Autodesk Inventor part; units mm, degrees
ref_plane "Work Plane2" through (-14.9733, -35.8014, 0) normal (0, 0, 1) x (1, 0, 0)
ref_plane "YZ Plane" through (0, 0, 0) normal (1, 0, 0) x (0, 1, 0)
ref_plane "XZ Plane" through (0, 0, 0) normal (0, 1, 0) x (-1, 0, 0)
ref_plane "Work Plane1" through (0, 0, 6.35) normal (0, 0, 1) x (1, 0, 0)
sketch "Sketch1" plane through (0, 0, 6.35) normal (0, 0, 1) x (1, 0, 0)
  line L0 (14.9733, -35.8014) -> (14.9733, 35.8014)
  line L1 (14.9733, 35.8014) -> (-14.9733, 35.8014)
  line L2 (-14.9733, 35.8014) -> (-14.9733, -35.8014)
  line L3 (-14.9733, -35.8014) -> (14.9733, -35.8014)
  circle A0 centre (-13.81, -28.5989) radius 0.6
  circle A1 centre (-11.557, -24.257) radius 0.1524
  circle A2 centre (-9.271, -23.749) radius 0.1524
  circle A3 centre (-8.636, -22.606) radius 0.1524
  circle A4 centre (-8.636, -19.939) radius 0.1524
  circle A5 centre (-6.731, -35.3061) radius 0.1524
  circle A6 centre (-5.842, -34.1631) radius 0.1524
  circle A7 centre (-7.239, -31.8771) radius 0.1524
  circle A8 centre (-5.08, -31.7501) radius 0.1524
  circle A9 centre (-5.08, -30.8611) radius 0.1524
  circle A10 centre (-1.016, -32.6391) radius 0.1524
  circle A11 centre (-1.905, -27.9401) radius 0.1524
  circle A12 centre (-4.318, -24.892) radius 0.1524
  circle A13 centre (-5.842, -19.05) radius 0.1524
  circle A14 centre (-5.08, -21.463) radius 0.1524
  circle A15 centre (-5.08, -18.415) radius 0.1524
  circle A16 centre (-4.191, -19.939) radius 0.1524
  circle A17 centre (-4.191, -18.415) radius 0.1524
  circle A18 centre (-11.176, -17.526) radius 0.1525
  circle A19 centre (-13.014, -12.8141) radius 1.016
  circle A20 centre (-7.874, -8.382) radius 1.85
  circle A21 centre (-4.826, -17.526) radius 0.1524
  circle A22 centre (-4.572, -5.715) radius 0.1524
  circle A23 centre (-2.413, -6.35) radius 0.1524
  circle A24 centre (-1.016, -5.715) radius 0.1524
  circle A25 centre (4.953, -31.4961) radius 0.1524
  circle A26 centre (6.35, -30.6071) radius 0.1524
  circle A27 centre (6.19, -28.5989) radius 0.85
  circle A28 centre (0.254, -24.638) radius 0.1524
  circle A29 centre (1.27, -21.082) radius 0.1524
  circle A30 centre (6.604, -26.2891) radius 0.1524
  circle A31 centre (5.461, -21.717) radius 0.1524
  circle A32 centre (8.509, -32.7661) radius 0.1524
  circle A33 centre (8.636, -30.6071) radius 0.1524
  circle A34 centre (12.986, -33.8141) radius 1.016
  circle A35 centre (13.843, -30.0991) radius 0.1524
  circle A36 centre (9.017, -24.892) radius 0.1524
  circle A37 centre (9.779, -22.86) radius 0.1524
  circle A38 centre (7.366, -21.717) radius 0.1524
  circle A39 centre (-0.014, -16.637) radius 0.255
  circle A40 centre (3.429, -7.62) radius 0.1524
  circle A41 centre (10.287, -16.9782) radius 0.1524
  circle A42 centre (10.033, -9.779) radius 0.1524
  circle A43 centre (13.843, -17.526) radius 0.1524
  circle A44 centre (-4.953, 11.303) radius 0.1524
  circle A45 centre (-13.014, 33.886) radius 1.016
  circle A46 centre (-3.8002, 24.494) radius 0.5
  circle A47 centre (-4.4502, 34.2441) radius 0.5
  circle A48 centre (-1.4001, 27.0939) radius 0.45
  circle A49 centre (0, 13.843) radius 0.1524
  circle A50 centre (3.8002, 24.494) radius 0.5
  circle A51 centre (1.4001, 27.0939) radius 0.45
  circle A52 centre (4.4502, 34.2441) radius 0.5
  circle A53 centre (12.986, 33.886) radius 1.016
  line L4 (-18.7833, -39.6114) -> (-18.7833, 39.6114)
  line L5 (-18.7833, 39.6114) -> (18.7833, 39.6114)
  line L6 (18.7833, 39.6114) -> (18.7833, -39.6114)
  line L7 (18.7833, -39.6114) -> (-18.7833, -39.6114)
  point P0 (0, 0)
  dimension "d1" = 3.81
extrude "Extrusion1" add sketch "Sketch1" along normal blind 3.175 contours L3 L2 L1 L0 | A0 | A1 | A2 | A3 | A4 | A5 | A6 | A7 | A8 | A9 | A10 | A11 | A12 | A13 | A14 | A15 | A16 | A17 | A18 | A19 | A20 | A21 | A22 | A23 | A24 | A25 | A26 | A27 | A28 | A29 | A30 | A31 | A32 | A33 | A34 | A35 | A36 | A37 | A38 | A39 | A40 | A41 | A42 | A43 | A44 | A45 | A46 | A47 | A48 | A49 | A50 | A51 | A52 | A53 | L4 L5 L6 L7
sketch "Sketch2" plane through (0, 0, 6.35) normal (0, 0, -1) x (-1, 0, 0)
  circle A0 centre (-12.986, -33.8141) radius 1.016
  circle A1 centre (-12.986, 33.886) radius 1.016
  circle A2 centre (13.014, 33.886) radius 1.016
  circle A3 centre (-12.986, -33.8141) radius 3.556
  circle A4 centre (-12.986, 33.886) radius 3.556
  circle A5 centre (13.014, 33.886) radius 3.556
  line L0 (-12.986, 33.886) -> (13.014, 33.886)
  line L1 (13.014, 33.886) -> (13.014, -33.8141)
  line L2 (13.014, -33.8141) -> (-12.986, -33.8141)
  line L3 (-12.986, -33.8141) -> (-12.986, 33.886)
  circle A6 centre (13.014, -12.8141) radius 1.016
  circle A7 centre (13.014, -12.8141) radius 3.556
  point P0 (0, 0)
  dimension "d4" = 7.112
  dimension "d5" = 7.112
  dimension "d6" = 7.112
  dimension "d32" = 7.112
ref_plane "Work Plane2" through (-14.9733, -35.8014, 0) normal (0, 0, 1) x (1, 0, 0)
extrude "Extrusion2" add sketch "Sketch2" along normal up to surface (6.35 mm away) contours L2 L3 A0 | L2 A3 L3 A0 | A0 L3 A3 L2 | A0 L3 L2 | L3 A1 L0 A4 | A4 L0 A1 L3 | A7 L1 A6 | L1 A6 A7 | L3 L0 A1 | A1 L0 L3 | A6 L1 | L1 A6 | L0 A2 L1 A5 | A5 L1 A2 L0 | L0 L1 A2 | A2 L1 L0
sketch "Sketch3" plane through (12.986, -33.8141, 0) normal (0, 0, -1) x (-1, 0, 0)
  circle A0 centre (0, 67.7) radius 1.016
  circle A1 centre (0, 0) radius 1.016
  circle A2 centre (26, 67.7) radius 1.016
  circle A3 centre (26, 21) radius 3.556
  point P0 (12.986, 33.8141)
hole "Hole1" at (12.986, -33.8141, 0) at (12.986, 33.886, 0) at (-13.014, 33.886, 0) at (-13.014, -12.8141, 0) direction (0, 0, 1) diameter 3.556 depth 6.35 countersink diameter 3.81 countersink angle 82
sketch "Sketch4" plane through (0, 0, 6.35) normal (0, 0, -1) x (-1, 0, 0)
  circle A0 centre (-12.986, 33.886) radius 3.556
  circle A1 centre (13.014, 33.886) radius 3.556
  circle A2 centre (-12.986, -33.8141) radius 3.556
  line L0 (18.7833, -39.6114) -> (-18.7833, -39.6114)
  line L1 (18.7833, 39.6114) -> (18.7833, -39.6114)
  line L2 (-18.7833, 39.6114) -> (18.7833, 39.6114)
  line L3 (-18.7833, -39.6114) -> (-18.7833, 39.6114)
  line L4 (-15.6083, 36.4364) -> (15.6083, 36.4364)
  line L5 (15.6083, 36.4364) -> (15.6083, -36.4364)
  line L6 (15.6083, -36.4364) -> (-15.6083, -36.4364)
  line L7 (-15.6083, -36.4364) -> (-15.6083, 36.4364)
  point P0 (0, 0)
  dimension "d17" = 3.175
extrude "Extrusion3" add sketch "Sketch4" along normal blind 21.59 contours L4 A0 | A0 L7 | A1 L4 | L7 A2 | L5 A1 | A2 L6 | L0 L3 L2 L1
sketch "Sketch5" plane through (-18.7833, 39.6114, 9.525) normal (0, 1, 0) x (1, 0, 0)
  line L0 (14.1836, 11.2166) -> (14.1836, 14.2664)
  line L1 (23.3831, 14.2664) -> (23.3831, 11.2166)
  line L2 (33.7567, 9.525) -> (33.7567, 11.125)
  line L3 (33.7567, 11.125) -> (3.81, 11.125)
  line L4 (3.81, 9.525) -> (3.81, 11.125)
  line L5 (33.7567, 9.525) -> (3.81, 9.525)
  line L6 (14.1836, 11.125) -> (23.3831, 11.125)
  line L7 (23.3831, 11.125) -> (23.3831, 17.475)
  line L8 (23.3831, 17.475) -> (14.1836, 17.475)
  line L9 (14.1836, 17.475) -> (14.1836, 11.125)
  point P0 (18.7833, 9.525)
  dimension "d20" = 6.35
extrude "Extrusion4" cut sketch "Sketch5" against normal up to surface (3.175 mm away) contours L0 L9 L8 L7 L1 L3
sketch "Sketch6" plane through (-18.7833, 39.6114, 9.525) normal (0, 1, 0) x (1, 0, 0)
  circle A0 centre (9.9291, 12.7125) radius 1.5875
  line L0 (14.1836, 11.125) -> (14.1836, 17.475)
  line L1 (23.3831, 11.125) -> (14.1836, 11.125)
  point P0 (18.7833, 9.525)
  dimension "d23" = 4.2545
  dimension "d24" = 3.175
  dimension "d25" = 1.5875
extrude "Extrusion5" cut sketch "Sketch6" against normal up to surface (3.175 mm away)
sketch "Sketch7" plane through (18.7833, -39.6114, 9.525) normal (1, 0, 0) x (0, 0, -1)
  circle A0 centre (20.6375, 72.6187) radius 1.905
  circle A1 centre (20.6375, 6.604) radius 1.778
  circle A2 centre (20.6375, 6.604) radius 1.905
  circle A3 centre (20.6375, 72.6187) radius 1.778
  circle A4 centre (20.6375, 72.6187) radius 1.016
  circle A5 centre (20.6375, 6.604) radius 1.016
  point P0 (9.525, 39.6114)
  dimension "d33" = 2.032
  dimension "d34" = 2.032
extrude "Extrusion6" cut sketch "Sketch7" against normal up to surface (37.5667 mm away) contours A4 | A5
properties part number "SENSOR_BOTTOM" material "PC/ABS Plastic"
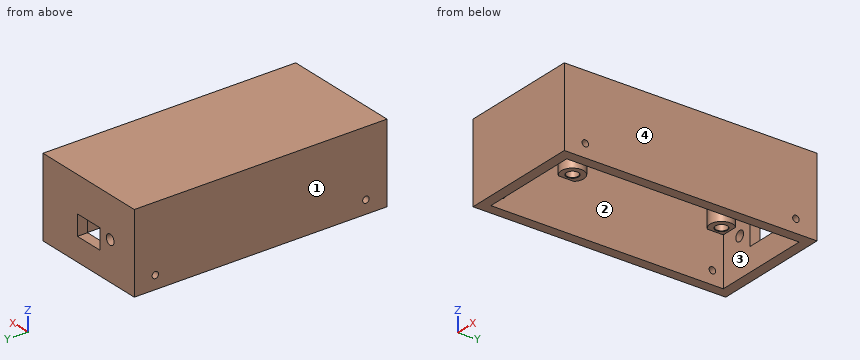
For this review, take the finished solid that the model builds, in its own axes (mm). Face numbers are marked on the shaded views. Round coordinates to 2 decimals unless told otherwise and drop trailing zeros. Order: outer loops, then holes, each group sorted by start corner. A loop starts at its lowest first (then second) coordinate and runs counter-clockwise, first axis right, second up. Notation, with made-up numbers: (-25.5, 10.25) -> (16.5, 10.25) arc R21 ccw to (16.5, 44.25) -> close; hole circle Ø8 at (18, 48.25). An arc over 180 degrees is marked (long way). Put each result on its own line as item: value.
Q1. For probe 1 along Y at (x, z) = (-11, -12.5); probe 2 along X at (y, z) = (-30, -1.5); probe 3 along Y at (x, z) = (-11, 2.75), list the stretches that pass through material, from the lowest coordinate up. Write a range as [from, to].
Check result:
probe 1: [-39.61, -36.44], [36.44, 39.61]
probe 2: [-18.78, -15.61], [15.61, 18.78]
probe 3: [-39.61, -36.44], [-15.74, -9.88], [30.96, 39.61]
Q2. Add section C-C on y = 15. Write out the cut boundary in (x, z) (3 decimals).
Check result:
outline: (-18.783, -15.24) -> (-15.608, -15.24) -> (-15.608, 6.35) -> (15.608, 6.35) -> (15.608, -15.24) -> (18.783, -15.24) -> (18.783, 9.525) -> (-18.783, 9.525) -> close
Q3. Mouldability with a two-part tool opening along X and no side actions: class the marked faces 1, 2, 3 and 4 as pulls with the +X half, pulls with the -X half, needs draft (parallel to the pull), parting line crosses it, or undercut.
Check result:
face 1: pulls with the -X half
face 2: undercut
face 3: undercut
face 4: pulls with the +X half
Q4. Add section D-D on z = 3.5. State how many separate pieces and enclosed holes the cut face has, plus the area to 3 significant figures.
Check result:
separate pieces: 1
enclosed holes: 8
area: 798 mm2
Q5. Add section A-A on x = -3. Write out the cut boundary in (y, z) (3 decimals).
Check result:
outline: (-39.611, -15.24) -> (-36.436, -15.24) -> (-36.436, 6.35) -> (36.436, 6.35) -> (36.436, -1.6) -> (39.611, -1.6) -> (39.611, 9.525) -> (-39.611, 9.525) -> close; (36.436, -15.24) -> (39.611, -15.24) -> (39.611, -7.95) -> (36.436, -7.95) -> close
Q6. Insertion check: pin 1 Ø4 at (x, y) = (-13.014, 33.886) entering from -Z; pin 2 Ø1.8 at (x, y) = (-13.5, 34.5) entering from -Z. Each pin has a flat end and moves straight along its axis. Give the tip position at first contact, or say it passes through.
Check result:
pin 1: z = 0
pin 2: z = 6.35
Q7. Add section B-B on z = -9.25. Write out the cut boundary in (x, y), plus the area to 3 significant figures.
Check result:
outline: (-18.78, -39.61) -> (18.78, -39.61) -> (18.78, 39.61) -> (-18.78, 39.61) -> close; hole (-15.61, -36.44) -> (15.61, -36.44) -> (15.61, 36.44) -> (-15.61, 36.44) -> close
area: 701 mm2
